Model file for the job. Use its own axes, mm. Coordinates: 2 decimals unless noted, no trailing zeros. Write each loop counter-clockwise with the first axis right and the second up, starting at its lowest first coordinate (ties: lowest second). Pieces come first, ordered by that corner, then holes. Notation, with made-up numbers: M 1.25,69.5 L 37.25,69.5 A30 ccw 37.25,96.5 Z; hole C -5,19 d3. An arc over 180 degrees is marked long. Put each result on its own line as item: value. Start each with the question number.
Q1. Cut at B-B (y = 16). Write the cut outline in (x, z), then the cut area to 3 significant figures.
Q2. Cut at C-C (x = 50.8). Write the cut outline in (y, z), then the cut area to 3 significant figures.
Q3. Drill centre lines: line 1 along Z through (x, y) = (50.8, 32.5); line 2 along X through (y, z) = (35, 25); line 3 along X through (y, z) = (38, 31). Where is each one in solid material? Low to high.
Q4. Cut at A-A (z = 25.4). Write the cut outline in (x, y).
Q5. Pull direction Z, two halves, no side cores. Call faces 1 (the cylindrical face through (56.666, 31.306, 22.968)), 2 (the flat face through (50, 32, 0)), 3 (the cylindrical face through (1.91, 61.69, 18.78)): pulls with the +Z half, pulls with the -Z half, needs draft (parallel to the pull), parting line crosses it, or undercut.
```python
from build123d import *

# Parameters (mm, degrees)
F1_DEPTH = 38.1
F2_R     = 6.35
F3_DEPTH = 63.501


with BuildPart() as f1:
    # F0 (on Top) → F1 (new body)
    with BuildSketch(Plane.XY):
        with BuildLine():
            ThreePointArc((0, 6.35), (1.859872, 1.859872), (6.35, 0))
            Line((6.35, 0), (95.25, 0))
            ThreePointArc((95.25, 0), (99.740128, 1.859872), (101.6, 6.35))
            Line((101.6, 6.35), (101.6, 57.15))
            ThreePointArc((101.6, 57.15), (99.740128, 61.640128), (95.25, 63.5))
            Line((95.25, 63.5), (6.35, 63.5))
            ThreePointArc((6.35, 63.5), (1.859872, 61.640128), (0, 57.15))
            Line((0, 57.15), (0, 6.35))
        make_face()
    extrude(amount=F1_DEPTH)

    # F2 (on face) → F3 (cut, through all)
    with BuildSketch(Plane.XZ):
        with Locations((50.8, 25.4)):
            Circle(F2_R)
    extrude(amount=-F3_DEPTH, mode=Mode.SUBTRACT)


solid = f1.part
```
Computed values:
1. outline: M 0,0 L 101.6,0 L 101.6,38.1 L 0,38.1 Z; hole C 50.8,25.4 d12.7
1. area: 3,740 mm2
2. outline: M 0,0 L 63.5,0 L 63.5,19.05 L 0,19.05 Z; M 0,31.75 L 63.5,31.75 L 63.5,38.1 L 0,38.1 Z
2. area: 1,610 mm2
3. line 1: 0 to 19.05, 31.75 to 38.1
3. line 2: 0 to 44.46, 57.14 to 101.6
3. line 3: 0 to 47.81, 53.79 to 101.6
4. outline: M 0,6.35 A6.35 ccw 6.35,0 L 44.45,0 L 44.45,63.5 L 6.35,63.5 A6.35 ccw 0,57.15 Z; M 57.15,0 L 95.25,0 A6.35 ccw 101.6,6.35 L 101.6,57.15 A6.35 ccw 95.25,63.5 L 57.15,63.5 Z
5. face 1: undercut
5. face 2: pulls with the -Z half
5. face 3: needs draft
